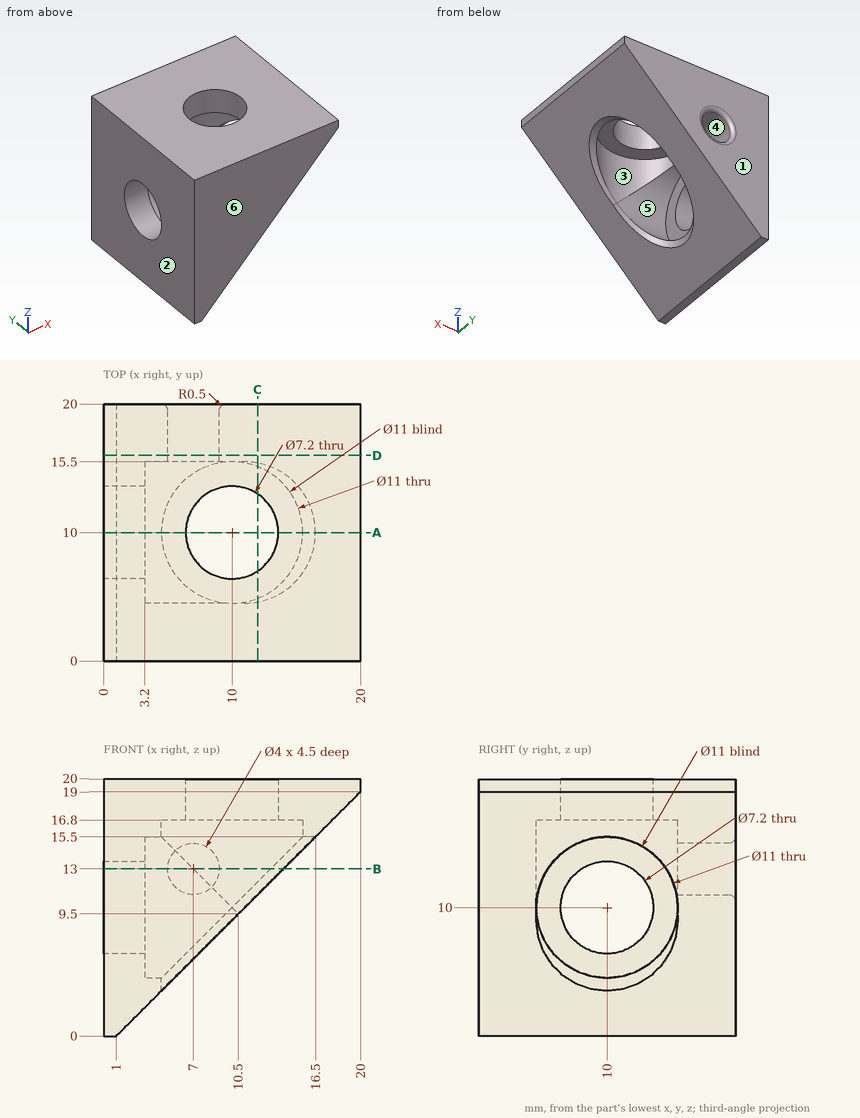
Geometry check sheet. Reference: drawing and pictorial views, mm from the part's lowest x, y, z. A direction names the side the tool comes from. Coordinates: 2 decimals unless noted, no trailing zeros. Write each loop counter-clockwise with the first axis right and the second up, starting at its lowest first coordinate (ties: lowest second). Pieces come first, ordered by that corner, then holes. Notation, with made-up numbers: M 28,81 L 72,81 A12 ccw 72,96 Z; hole C -15.5,-15.75 d10. An arc over 180 degrees is marked long. Write item = value, one per line. Start each with the question number.
1. Thickness scan on probe 1 along Y at (x, z) = (7.75, 10); probe 2 along Z at (x, y) = (6.5, 6.5); probe 3 along Z at (x, y) = (4.5, 14). Record the ranges inside material, lowest first.
2. Sectioned sample at A-A (y = 10). Record the cut outline in (x, z), then the cut area to 3 significant figures.
3. Tool access check on the marked faces 4, 5 and 6. Record the directions out of +Z, -Z, +X, -X, +Y, -Y that give a thin tool (end or side, any length) a straight path to the whole face; none if there is none.
4. Mould release check, pull along X, two halves, no side actions. Record for the marked faces 1, 2 and 3: pulls with the +X half, pulls with the -X half, needs draft (parallel to the pull), parting line crosses it, or undercut.
5. Sectioned sample at C-C (x = 12). Record the cut outline in (y, z).
6. Go/stop test with flat-tipped pins: pin 1 (2 mm diameter, centred on x = 7, z = 13.5, fed in from +Y); pin 2 (9.5 mm diameter, centred on x = 10, y = 10, fed in from -Z); pin 3 (5.5 mm diameter, centred on y = 11.5, z = 9.5, fed in from +X). Record where each tip stops, or that it passes through.
7. Sectioned sample at B-B (z = 13). Record the cut outline in (x, y).
8. Sectioned sample at D-D (y = 16). Record the cut outline in (x, z).
The answers:
q1.probe_1 = 0 to 4.5, 15.5 to 20
q1.probe_2 = 16.8 to 20
q1.probe_3 = 3.5 to 6.23, 13.77 to 20
q2.outline = M 0,0 L 1,0 L 4.5,3.5 L 4.5,4.5 L 3.2,4.5 L 3.2,6.4 L 0,6.4 Z; M 0,13.6 L 3.2,13.6 L 3.2,15.5 L 4.5,15.5 L 4.5,16.8 L 6.4,16.8 L 6.4,20 L 0,20 Z; M 13.6,16.8 L 15.5,16.8 L 15.5,15.5 L 16.5,15.5 L 20,19 L 20,20 L 13.6,20 Z
q2.area = 72.8 mm²
q3.face_4 = +Y
q3.face_5 = +X
q3.face_6 = +Z, -Z, +X, -X, -Y
q4.face_1 = needs draft
q4.face_2 = pulls with the -X half
q4.face_3 = undercut
q5.outline = M 0,11 L 4.59,11 A5.5 cw 4.88,12 L 4.88,16.8 L 7.01,16.8 L 7.01,20 L 0,20 Z; M 12.99,16.8 L 15.12,16.8 L 15.12,12 A5.5 cw 15.41,11 L 20,11 L 20,20 L 12.99,20 Z
q6.pin_1 = 15.5
q6.pin_2 = 16.8
q6.pin_3 = 3.2
q7.outline = M 0,0 L 14,0 L 14,5.39 L 13,5.39 A5.5 cw 7,5.39 L 3.2,5.39 L 3.2,8.01 L 0,8.01 Z; M 0,11.99 L 3.2,11.99 L 3.2,14.61 L 7,14.61 A5.5 cw 13,14.61 L 14,14.61 L 14,20 L 9.5,20 A0.5 ccw 9,19.5 L 9,15.5 L 5,15.5 L 5,19.5 A0.5 ccw 4.5,20 L 0,20 Z
q8.outline = M 0,0 L 1,0 L 20,19 L 20,20 L 0,20 Z; hole C 7,13 d4
